from build123d import *

# Parameters (mm, degrees)
SKETCH6_W           = 1000
SKETCH6_H           = 40
BOSS_EXTRUDE3_DEPTH = 40
SKETCH7_W           = 15
SKETCH7_H           = 23
CUT_EXTRUDE3_DEPTH  = 1064
CUT_EXTRUDE4_DEPTH  = 1064


with BuildPart() as part:
    # Sketch6 → Boss-Extrude3 (new body)
    with BuildSketch(Plane.XY):
        with Locations((439.141785032, 79.78108724)):
            Rectangle(SKETCH6_W, SKETCH6_H)
    extrude(amount=BOSS_EXTRUDE3_DEPTH)

    # Sketch7 → Cut-Extrude3 (cut)
    with BuildSketch(Plane.ZY.offset(60.858214968)):
        with Locations((32.5, 86.28108724)):
            Rectangle(SKETCH7_W, SKETCH7_H)
        Polygon((25, 74.78108724), (2, 74.78108724), (2, 59.78108724), (40, 59.78108724), (40, 74.78108724), align=None)
    extrude(amount=-CUT_EXTRUDE3_DEPTH, mode=Mode.SUBTRACT)

    # Sketch8 → Cut-Extrude4 (cut)
    with BuildSketch(Plane(origin=(0, 0, 0), x_dir=(-1, 0, 0), z_dir=(0, 0, -1))):
        Polygon((-939.141785032, 99.78108724), (-899.141785032, 59.78108724), (-939.141785032, 59.78108724), align=None)
        Polygon((60.858214968, 59.78108724), (20.858214968, 59.78108724), (60.858214968, 99.78108724), align=None)
    extrude(amount=-CUT_EXTRUDE4_DEPTH, mode=Mode.SUBTRACT)


solid = part.part
Model file for the job. Use its own axes, mm. A direction names the side the tool comes from. Round coordinates to 2 decimals unless told otherwise and drop trailing zeros. Loops run counter-clockwise (first coordinate to the right, second up) from the corner with the lowest first, then second, coordinate; pieces in that order, holes last. Notation, with made-up numbers: M 87.5,-12 L 130.5,-12 A29 ccw 130.5,21 Z; hole C 6.5,58.25 d10. An arc over 180 degrees is marked long. One line per question, with ' | ' between items.
1) 3-axis set-ups, long thin cutter, end or side, ignore diameter. For faces 1 (the flat face through (432, 74.781, 14)), 2 (the flat face through (432, 80, 0)): which of +Z, -Z, +X, -X, +Y, -Y reach the whole face in a straight line?
Solved:
face 1: +Z, +X, -X, -Y | face 2: -Z, +X, -X, +Y, -Y
2) Band-saw the part on B-B (z = 31). Give the cut face in (x, y), then the cut area to 3 significant figures.
Solved:
outline: M -60.86,99.78 L -58.86,97.78 L 937.14,97.78 L 939.14,99.78 Z | area: 2,000 mm²
3) Band-saw the part on A-A (x = 416). Give the cut face in (y, z), then the cut area to 3 significant figures.
Solved:
outline: M 59.78,0 L 99.78,0 L 99.78,40 L 97.78,40 L 97.78,25 L 74.78,25 L 74.78,2 L 59.78,2 Z | area: 685 mm²
4) Mould opens along Y. For faces 3 (the flat face through (432, 86, 25)), 4 (the flat face through (432, 99.781, 20)), 5 (the flat face through (923.87, 84.51, 15.28)) say: +Y half, -Y half, draft (parallel to the pull), parting line (faces both ways), or undercut.
Solved:
face 3: draft | face 4: +Y half | face 5: -Y half
5) Band-saw the part on C-C (y = 82). Give the cut face in (x, z).
Solved:
outline: M -43.08,0 L 921.36,0 L 921.36,25 L -43.08,25 Z
6) Flat gauge pins, fed straight in: pin 1 (4.5 mm diameter, centred on x = 526.5, z = 31.5, fed in from -Y); pin 2 (10 mm diameter, centred on y = 67, z = 13, fed in from +X); pin 3 (18.5 mm diameter, centred on x = 274, y = 83.5, fed in from +Z); pin 4 (8 mm diameter, centred on x = 532, z = 25, fed in from -Y). Where does each tip first touch, or does it go through?
Solved:
pin 1: stops at y = 97.78 | pin 2: passes through | pin 3: stops at z = 25 | pin 4: stops at y = 74.78
7) Drill centre lines: line 1 along Z through (x, y) = (770, 90); line 2 along Y through (x, z) = (828, 26.5); line 3 along Y through (x, z) = (845, 21.5). Where is each one in solid material? Low to high.
Solved:
line 1: z = 0 to 25 | line 2: y = 97.78 to 99.78 | line 3: y = 74.78 to 99.78
